Design review of the part built by this model. Coordinates are the model's own, in mm. A direction names the side the tool comes from. Coordinates: 2 decimals unless noted, no trailing zeros. Write each loop counter-clockwise with the first axis right and the second up, starting at its lowest first coordinate (ties: lowest second). Pieces come first, ordered by that corner, then holes. Notation, with made-up numbers: (3.25, -17) - (12.25, -17) arc R9 cw to (12.25, -5) - close; hole circle Ø9 at (65, 15.5). An arc over 180 degrees is marked (long way). Answer as a JSON object with one key per item and string values.
```python
from build123d import *

# Parameters (mm, degrees)
SKETCH1_W           = 431.8
SKETCH1_H           = 457.2
BOSS_EXTRUDE1_DEPTH = 685.8
SKETCH2_W           = 431.8
SKETCH2_H           = 533.4
BOSS_EXTRUDE2_DEPTH = 812.8
BOSS_EXTRUDE4_DEPTH = 660.4
BOSS_EXTRUDE3_DEPTH = 660.4
CUT_EXTRUDE3_DEPTH  = 76.2
SKETCH7_R           = 25.4
BOSS_EXTRUDE5_DEPTH = 19.05
CHAMFER1_SIZE       = 13.335
CHAMFER1_SIZE2      = 23.096897519
SKETCH8_R           = 1.5875
SKETCH8_R_2         = 0.635
BOSS_EXTRUDE6_DEPTH = 2.54


with BuildPart() as part:
    # Sketch1 → Boss-Extrude1 (new body)
    with BuildSketch(Plane(origin=(0, 0, 0), x_dir=(1, 0, 0), z_dir=(0, 1, 0))):
        Rectangle(SKETCH1_W, SKETCH1_H)
    extrude(amount=BOSS_EXTRUDE1_DEPTH)

    # Sketch2 → Boss-Extrude2 (add)
    with BuildSketch(Plane(origin=(0, 0, 0), x_dir=(1, 0, 0), z_dir=(0, 1, 0))):
        with Locations((-431.8, -38.1)):
            Rectangle(SKETCH2_W, SKETCH2_H)
    extrude(amount=BOSS_EXTRUDE2_DEPTH)

    # Sketch4 → Boss-Extrude4 (add)
    with BuildSketch(Plane(origin=(0, 0, 0), x_dir=(1, 0, 0), z_dir=(0, 1, 0))):
        with BuildLine():
            Line((-152.4, -251.46), (-152.4, -228.6))
            Line((-152.4, -228.6), (215.9, -228.6))
            ThreePointArc((215.9, -228.6), (32.104383146, -245.739506237), (-152.4, -251.46))
        make_face()
    extrude(amount=BOSS_EXTRUDE4_DEPTH)

    # Sketch3 → Boss-Extrude3 (add)
    with BuildSketch(Plane(origin=(0, 0, 0), x_dir=(1, 0, 0), z_dir=(0, 1, 0))):
        with BuildLine():
            Line((-279.4, -304.8), (-279.4, -327.66))
            ThreePointArc((-279.4, -327.66), (-463.904383146, -321.939506237), (-647.7, -304.8))
            Line((-647.7, -304.8), (-279.4, -304.8))
        make_face()
    extrude(amount=BOSS_EXTRUDE3_DEPTH)

    # Sketch6 → Cut-Extrude3 (cut)
    with BuildSketch(Plane.XY.offset(304.8)):
        with BuildLine():
            Line((33.909716126, 248.55832752), (82.654926159, 491.804601993))
            ThreePointArc((82.654926159, 491.804601993), (80.025469047, 502.349796436), (70.202497127, 507))
            Line((70.202497127, 507), (-102.002497127, 507))
            ThreePointArc((-102.002497127, 507), (-111.825469047, 502.349796436), (-114.454926159, 491.804601993))
            Line((-114.454926159, 491.804601993), (-65.709716126, 248.55832752))
            ThreePointArc((-65.709716126, 248.55832752), (-15.9, 207.739919548), (33.909716126, 248.55832752))
        make_face()
    extrude(amount=-CUT_EXTRUDE3_DEPTH, mode=Mode.SUBTRACT)



with BuildPart() as body_2:
    # Sketch7 → Boss-Extrude5 (new body)
    with BuildSketch(Plane.XY.offset(228.6)):
        with Locations(Location((-15.9, 380, 0), (0, 0, 180))):
            Circle(SKETCH7_R)
    extrude(amount=BOSS_EXTRUDE5_DEPTH)

    # Chamfer1
    chamfer1_edges = [body_2.edges().sort_by_distance(p)[0] for p in [
        (9.5, 380, 247.65),
    ]]
    chamfer1_side = [body_2.faces().sort_by_distance(p)[0] for p in [
        (9.5, 380, 238.125),
    ]]
    chamfer(chamfer1_edges, length=CHAMFER1_SIZE, length2=CHAMFER1_SIZE2, reference=chamfer1_side[0])


with BuildPart() as part_1:
    add(part.part)

    add(body_2.part)  # Boss-Extrude6 merges body 2
    # Sketch8 → Boss-Extrude6 (add)
    with BuildSketch(Plane.XY.offset(247.65)):
        with Locations((-15.9, 380)):
            Circle(SKETCH8_R)
        with Locations((-15.9, 380)):
            Circle(SKETCH8_R_2, mode=Mode.SUBTRACT)
    extrude(amount=BOSS_EXTRUDE6_DEPTH)


solid = part_1.part
```
(1) Take a section at A-A, the plane y = 550. Write out the cut boundary in (x, z).
Solved:
{"outline": "(-647.7, -228.6) - (215.9, -228.6) - (215.9, 228.6) arc R2978.29 ccw to (-152.4, 251.46) - (-152.4, 228.6) - (-215.9, 228.6) - (-215.9, 304.8) - (-279.4, 304.8) - (-279.4, 327.66) arc R2978.29 ccw to (-647.7, 304.8) - close"}
(2) Take a section at D-D, the plane y = 324.5. Write out the cut boundary in (x, z), and give its area (3 significant figures).
Solved:
{"outline": "(-647.7, -228.6) - (215.9, -228.6) - (215.9, 228.6) arc R2978.29 ccw to (49.13, 244.63) - (49.13, 228.6) - (-80.93, 228.6) - (-80.93, 250.6) arc R2978.29 ccw to (-152.4, 251.46) - (-152.4, 228.6) - (-215.9, 228.6) - (-215.9, 304.8) - (-279.4, 304.8) - (-279.4, 327.66) arc R2978.29 ccw to (-647.7, 304.8) - close", "area": "436,000 mm^2"}
(3) Tool access review of faces 1 (the face through (-39, 393, 228.6)), 2 (the face through (-420, 660.4, 314)), 3 (the face through (-279.4, 326, 316)): name each direction out of +Z, -Z, +X, -X, +Y, -Y from which nothing blocks a thin tool from reaching the whole face with its end or side.
Solved:
{"face 1": "+Z", "face 2": "+Z, +X, -X, +Y", "face 3": "+Z, +X, +Y, -Y"}
(4) Take a section at B-B, the plane z = 129.5. Write out the cut boundary in (x, y).
Solved:
{"outline": "(-647.7, 0) - (215.9, 0) - (215.9, 685.8) - (-215.9, 685.8) - (-215.9, 812.8) - (-647.7, 812.8) - close"}
(5) For pin 1 (1.4 mm diameter, centred on x = -16, y = 380, fed in from +Z); pin 2 (18.5 mm diameter, centred on x = -40.5, z = 243.5, fed in from +Y); pin 3 (11.5 mm diameter, centred on y = 441.5, z = 317, fed in from +X), all flat-tipped, find the tip position at first contact; note any pin that passes through.
Solved:
{"pin 1": "stops at z = 250.19", "pin 2": "stops at y = 660.4", "pin 3": "stops at x = -279.4"}
(6) Take a section at C-C, the plane x = -574. Write out the cut boundary in (y, z).
Solved:
{"outline": "(0, -228.6) - (812.8, -228.6) - (812.8, 304.8) - (660.4, 304.8) - (660.4, 313.05) - (0, 313.05) - close"}
(7) The part is to be moulded in two halves that separate along Y. For faces 4 (the face through (-222, 401, -228.6)), 5 (the face through (-7, 660.4, 237)), 6 (the face through (-10.394, 404.796, 231.417)), say which applies: pulls with the +Y half, pulls with the -Y half, needs draft (parallel to the pull), parting line crosses it, or undercut.
Solved:
{"face 4": "needs draft", "face 5": "pulls with the +Y half", "face 6": "undercut"}
(8) To check wall thickness, follow line 1 (X direction, y = 380, z = 249.35) (1 decimal); line 2 (Y direction, x = -15.9, z = 248.9) (1 decimal); line 3 (Z direction, x = -156, y = 41). State the ranges of each line that lie inside material, in increasing order. Write a range as from..to.
Solved:
{"line 1": "x = -647.7..-215.9, -152.4..-92, -17.5..-16.5, -15.3..-14.3", "line 2": "y = 378.4..379.4, 380.6..381.6", "line 3": "z = -228.6..228.6"}
